Could you check a few things on this drawing? It's one solid part, dimensions in mm from its lowest x, y, z. A direction names the side the tool comes from. Give positions to 0.01 mm unless a question says otherwise; leave off trailing zeros. Order: outer loops, then holes, each group sorted by start corner. A loop starts at its lowest first (then second) coordinate and runs counter-clockwise, first axis right, second up.
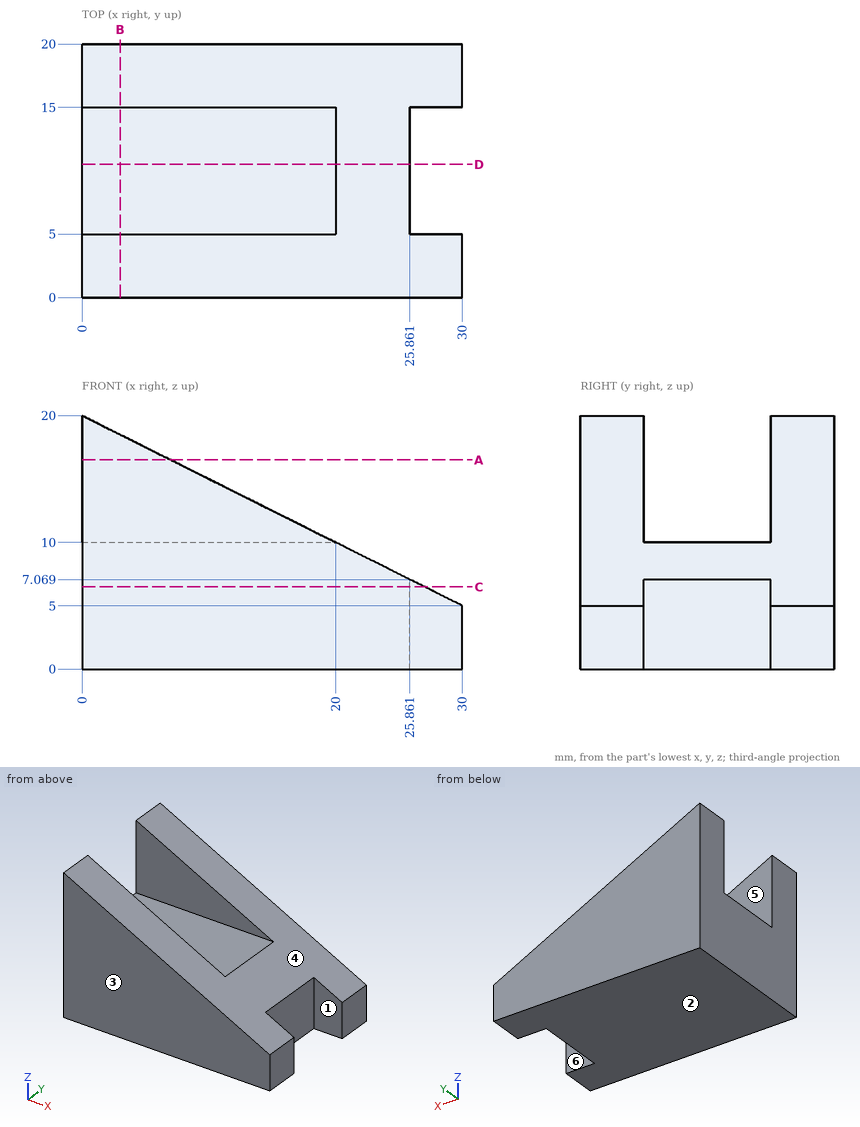
1) Suppose I cut it at B-B (x = 3). Please give me the cut outline in (y, z), and give its area (3 significant figures).
2) Suppose I cut it at D-D (y = 10.5). Please give me the cut outline in (x, z), and give its area (3 significant figures).
3) Suppose I cut it at C-C (z = 6.5). Please give me the cut outline in (x, y).
4) I'm going to push flat-ended pins straight in: pin 1 Ø2 at (x, y) = (5, 16) entering from +Z; pin 2 Ø10 at (x, y) = (13, 14.5) entering from +Z; pin 3 Ø5 at (x, y) = (7, 9) entering from +Z. Where does each tip first touch, or does it pass through?
5) Suppose I cut it at A-A (z = 16.5). Please give me the cut outline in (x, y), and give its area (3 significant figures).
6) If I drill on line 1 (Y direction, x = 4.5, z = 16.5); line 2 (Z direction, x = 5, y = 7.75); line 3 (X direction, y = 14.5, z = 2), over which ranges is the centre line in solid material (lowest first)?
7) We'd pull the mould along Y, two halves only. Please class the marked faces 1, 2 and 3: +Y half, -Y half, draft (parallel to the pull), parting line (faces both ways), or undercut.
8) Which directions (+Z, -Z, +X, -X, +Y, -Y) give clear straight access to the entire face, cutting with the end or side of a thin tool? Please do the marked faces 4, 5 and 6.
Results:
1. outline: (0, 0) - (20, 0) - (20, 18.5) - (15, 18.5) - (15, 10) - (5, 10) - (5, 18.5) - (0, 18.5) - close
1. area: 285 mm2
2. outline: (0, 0) - (25.86, 0) - (25.86, 7.07) - (20, 10) - (0, 10) - close
2. area: 250 mm2
3. outline: (0, 0) - (27, 0) - (27, 5) - (25.86, 5) - (25.86, 15) - (27, 15) - (27, 20) - (0, 20) - close
4. pin 1: stops at z = 18
4. pin 2: stops at z = 15.99
4. pin 3: stops at z = 10
5. outline: (0, 0) - (7, 0) - (7, 5) - (0, 5) - close; (0, 15) - (7, 15) - (7, 20) - (0, 20) - close
5. area: 70.0 mm2
6. line 1: y = 0 to 5, 15 to 20
6. line 2: z = 0 to 10
6. line 3: x = 0 to 25.86
7. face 1: undercut
7. face 2: draft
7. face 3: -Y half
8. face 4: +Z, +X, +Y, -Y
8. face 5: +Z, +X, -X
8. face 6: +Z, -Z, +X
